```python
from build123d import *

# Parameters (mm, degrees)
BOSS_EXTRUDE1_DEPTH = 7
BOSS_EXTRUDE2_DEPTH = 3
CUT_EXTRUDE1_DEPTH  = 14.62


with BuildPart() as part:
    # Sketch1 → Boss-Extrude1 (new body)
    with BuildSketch(Plane(origin=(0, 0, 0), x_dir=(0, 0, -1), z_dir=(1, 0, 0))):
        with BuildLine():
            ThreePointArc((2.69, 5.91), (1.902117241, 7.812117241), (0, 8.6))
            Line((0, 8.6), (0, 0))
            Line((0, 0), (0, -2.87))
            Line((0, -2.87), (7.31, -2.87))
            Line((7.31, -2.87), (7.31, 0))
            Line((7.31, 0), (4.31, 0))
            ThreePointArc((4.31, 0), (3.164487014, 0.474487014), (2.69, 1.62))
            Line((2.69, 1.62), (2.69, 5.91))
        make_face()
    boss_extrude1 = extrude(amount=-BOSS_EXTRUDE1_DEPTH)

    # Sketch1<3> → Boss-Extrude2 (add)
    with BuildSketch(Plane(origin=(0, 0, 0), x_dir=(0, 0, -1), z_dir=(1, 0, 0))):
        with BuildLine():
            Line((7.31, 10.1), (0, 10.1))
            Line((0, 10.1), (0, 8.6))
            ThreePointArc((0, 8.6), (1.902117241, 7.812117241), (2.69, 5.91))
            Line((2.69, 5.91), (2.69, 1.62))
            ThreePointArc((2.69, 1.62), (3.164487014, 0.474487014), (4.31, 0))
            Line((4.31, 0), (7.31, 0))
            Line((7.31, 0), (7.31, 10.1))
        make_face()
    boss_extrude2 = extrude(amount=-BOSS_EXTRUDE2_DEPTH)

    # Mirror1: Boss-Extrude1, Boss-Extrude2 across plane
    add(boss_extrude1.mirror(Plane.XY))
    add(boss_extrude2.mirror(Plane.XY))

    # Sketch2 → Cut-Extrude1 (cut)
    with BuildSketch(Plane(origin=(0, 0, -7.31), x_dir=(-1, 0, 0), z_dir=(0, 0, -1))):
        with BuildLine():
            Line((3, 10.1), (1.5, 10.1))
            ThreePointArc((1.5, 10.1), (2.560660172, 9.660660172), (3, 8.6))
            Line((3, 8.6), (3, 10.1))
        make_face()
    extrude(amount=-CUT_EXTRUDE1_DEPTH, mode=Mode.SUBTRACT)


solid = part.part
```
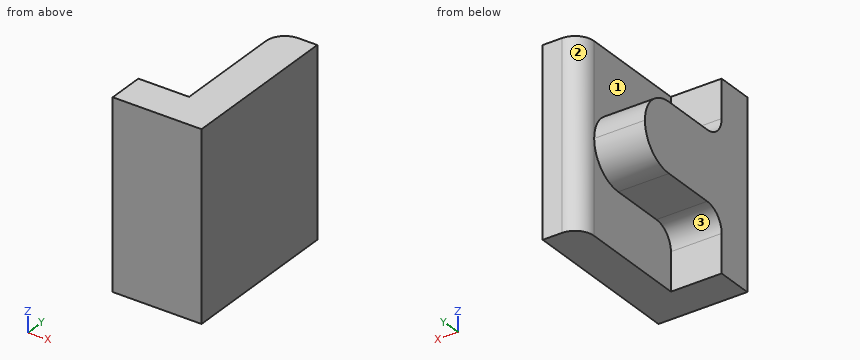
The model under review builds one solid part; all positions refer to its coordinate system, in mm. Face numbers are marked on the shaded views. A direction names the side the tool comes from. Coordinates: 2 decimals unless noted, no trailing zeros. Write each loop counter-clockwise with the first axis right and the second up, starting at its lowest first coordinate (ties: lowest second). Pieces come first, ordered by that corner, then holes. Notation, with made-up numbers: (84, 77) - (143, 77) arc R16 cw to (143, 97) - close; hole circle Ø4 at (1.5, 62). An arc over 180 degrees is marked (long way). Answer in a Markdown table with one row per item. Add a question column.
Q1. For the marked faces 1, 2 and 3, list the 3-axis set-ups (+Z, -Z, +X, -X, +Y, -Y) from which the entire face can be reached by the end or side of a thin tool; tool diameter is ignored.
Q2. Consider section C-C on x = -4. Give the boundary of the cut face in (y, z), then the cut area to 3 significant figures.
Q3. Consider section A-A on z = -5. Give the boundary of the cut face in (x, y), then the cut area to 3 significant figures.
Q4. Consider section B-B on y = 3.5. Give the boundary of the cut face in (x, z), then the cut area to 3 significant figures.
Q5. Clearance check with flat-ended pins moving along their axes: pin 1 (1.5 mm diameter, centred on x = -4.5, z = 5.5, fed in from +Y); pin 2 (2 mm diameter, centred on x = -5.5, y = 5, fed in from +Z); pin 3 (3.5 mm diameter, centred on y = 5, z = -4.5, fed in from -X). State where each tip first meets the part, or that it passes through.
Q6. To check wall thickness, follow line 1 along X through (y, z) = (4.25, -5.75); line 2 along Y through (x, z) = (-5.75, 6.5); line 3 along Z through (x, y) = (-4.25, 5). State the ranges of each line that lie inside material, in increasing order. Write a range as from..to.
Q7. Consider section D-D on z = -1.75. Give the boundary of the cut face in (x, y).
Answers below:
| question | item | result |
|---|---|---|
| 1 | face 1 | +Z, -X, +Y |
| 1 | face 2 | +Z, -Z, -X, +Y |
| 1 | face 3 | -Z, -X, +Y |
| 2 | outline | (-2.87, -7.31) - (0, -7.31) - (0, -4.31) arc R1.62 cw to (1.62, -2.69) - (5.91, -2.69) arc R2.69 ccw to (5.91, 2.69) - (1.62, 2.69) arc R1.62 cw to (0, 4.31) - (0, 7.31) - (-2.87, 7.31) - close |
| 2 | area | 86.2 mm² |
| 3 | outline | (-7, -2.87) - (0, -2.87) - (0, 10.1) - (-1.5, 10.1) arc R1.5 ccw to (-3, 8.6) - (-3, 0) - (-7, 0) - close |
| 3 | area | 49.9 mm² |
| 4 | outline | (-7, -2.69) - (-3, -2.69) - (-3, -7.31) - (0, -7.31) - (0, 7.31) - (-3, 7.31) - (-3, 2.69) - (-7, 2.69) - close |
| 4 | area | 65.4 mm² |
| 5 | pin 1 | y = 0 |
| 5 | pin 2 | z = 2.69 |
| 5 | pin 3 | x = -3 |
| 6 | line 1 | -3..0 |
| 6 | line 2 | -2.87..0 |
| 6 | line 3 | -2.69..2.69 |
| 7 | outline | (-7, -2.87) - (0, -2.87) - (0, 10.1) - (-1.5, 10.1) arc R1.5 ccw to (-3, 8.6) - (-3, 7.95) - (-7, 7.95) - close |
